Can you work these out from the drawing? Everything is in mm from the part's minimum corner. A direction names the side the tool comes from. Coordinates: 2 decimals unless noted, no trailing zeros. Loops run counter-clockwise (first coordinate to the right, second up) from the corner with the lowest first, then second, coordinate; pieces in that order, holes last.
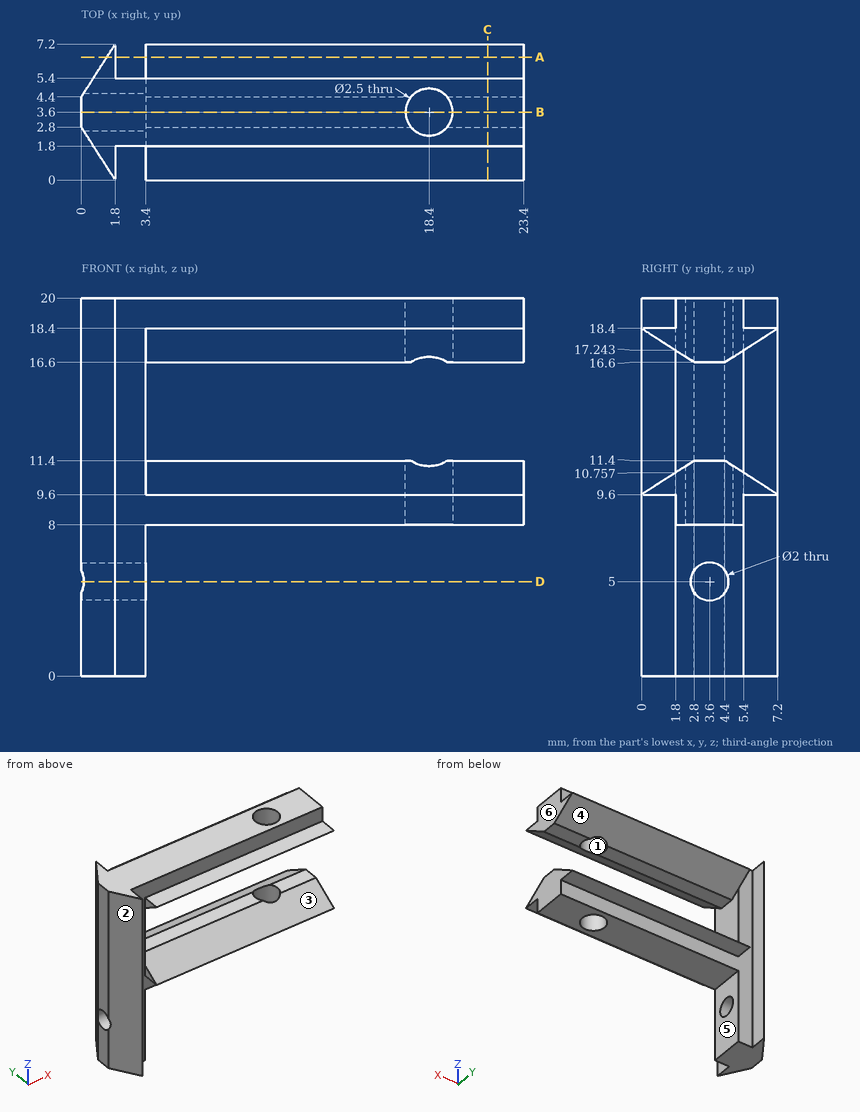
Item 1: On a 3-axis mill with a long thin cutter (end or side, diameter ignored), from which of +Z, -Z, +X, -X, +Y, -Y can I reach the whole of each face in a straight line? I mean the marked faces 4, 5 and 6. Say none if no direction works.
Results are:
face 4: +X, +Y
face 5: -Z, +X, +Y, -Y
face 6: +Z, -Z, +X, +Y, -Y
Item 2: I'm going to push flat-ended pins straight in: P1, Ø1.5, axis at x = 16, z = 16.5, coming from the -Y side; P2, Ø1.1, axis at x = 16, y = 3, coming from the -Z side; P3, Ø1, axis at x = 4.5, z = 11, coming from the +Y side. Where does each tip first touch, or does it pass through?
Results are:
P1: stops at y = 1.79
P2: stops at z = 8
P3: stops at y = 5.8
Item 3: Suppose I cut it at B-B, the plane y = 3.6. Please give me the cut outline in (x, z).
Results are:
outline: (0, 0) - (3.4, 0) - (3.4, 4) - (0, 4) - close; (0, 6) - (3.4, 6) - (3.4, 8) - (17.15, 8) - (17.15, 11.4) - (3.4, 11.4) - (3.4, 16.6) - (17.15, 16.6) - (17.15, 20) - (0, 20) - close; (19.65, 8) - (23.4, 8) - (23.4, 11.4) - (19.65, 11.4) - close; (19.65, 16.6) - (23.4, 16.6) - (23.4, 20) - (19.65, 20) - close
Item 4: I need wall thicknesses on line 1 along Z through (x, y) = (1.6, 3.6); line 2 along Z through (x, y) = (11.25, 3); line 3 along X through (y, z) = (3.5, 10.5). Which ranges of each line are inside material? Lowest first, please.
Results are:
line 1: z = 0 to 4, 6 to 20
line 2: z = 8 to 11.4, 16.6 to 20
line 3: x = 0 to 17.15, 19.65 to 23.4
Item 5: We'd pull the mould along X, two halves only. Please class the marked faces 1, 2 and 3: +X half, -X half, draft (parallel to the pull), parting line (faces both ways), or undercut.
Results are:
face 1: undercut
face 2: -X half
face 3: draft
Item 6: Suppose I cut it at C-C, the plane x = 21.5. Please give me the cut outline in (y, z).
Results are:
outline: (0, 9.6) - (1.8, 9.6) - (1.8, 8) - (5.4, 8) - (5.4, 9.6) - (7.2, 9.6) - (4.4, 11.4) - (2.8, 11.4) - close; (0, 18.4) - (2.8, 16.6) - (4.4, 16.6) - (7.2, 18.4) - (5.4, 18.4) - (5.4, 20) - (1.8, 20) - (1.8, 18.4) - close
Item 7: Suppose I cut it at D-D, the plane z = 5. Please give me the cut outline in (x, y).
Results are:
outline: (0.13, 2.6) - (1.8, 0) - (1.8, 1.8) - (3.4, 1.8) - (3.4, 2.6) - close; (0.13, 4.6) - (3.4, 4.6) - (3.4, 5.4) - (1.8, 5.4) - (1.8, 7.2) - close
Item 8: Suppose I cut it at A-A, the plane y = 6.5. Please give me the cut outline in (x, z).
Results are:
outline: (1.35, 0) - (1.8, 0) - (1.8, 20) - (1.35, 20) - close; (3.4, 9.6) - (23.4, 9.6) - (23.4, 10.05) - (3.4, 10.05) - close; (3.4, 17.95) - (23.4, 17.95) - (23.4, 18.4) - (3.4, 18.4) - close
